from build123d import *

# Parameters (mm, degrees)
SKETCH_1_R               = 87.5
SKETCH_1_R_2             = 70
EXTRUDE_1_DEPTH          = 8
SKETCH_2_R               = 2.75
CUT_EXTRUDE_1_DEPTH      = 10
PATTERN_CIRCULAR_1_COUNT = 4
EXTRUDE_START            = -8
SKETCH_3_R               = 2.75
EXTRUDE_2_DEPTH          = 8
PATTERN_CIRCULAR_2_COUNT = 4
FILLET_1_R               = 10


with BuildPart() as part:
    # 草图1 → 凸台-拉伸1 (new body)
    with BuildSketch(Plane.XY):
        Circle(SKETCH_1_R)
        Circle(SKETCH_1_R_2, mode=Mode.SUBTRACT)
    extrude(amount=EXTRUDE_1_DEPTH)

    # 草图2 → 切除-拉伸1 (cut)
    with BuildSketch(Plane.XY.offset(8)):
        with Locations((42.051550898, 69.52143243)):
            Circle(SKETCH_2_R)
        with Locations((53.351997363, 61.27909005)):
            Circle(SKETCH_2_R)
        with Locations((71.178427561, 39.181551143)):
            Circle(SKETCH_2_R)
        with Locations((15.564640034, 79.745247386)):
            Circle(SKETCH_2_R)
    cut_extrude_1 = extrude(amount=-CUT_EXTRUDE_1_DEPTH, mode=Mode.SUBTRACT)

    # 阵列(圆周)1: 切除-拉伸1 ×4 about axis
    pattern_circular_1_axis = Axis((0, 0, 0), (0, 0, 1))
    for i in range(1, PATTERN_CIRCULAR_1_COUNT):
        add(cut_extrude_1.rotate(pattern_circular_1_axis, i * 360 / PATTERN_CIRCULAR_1_COUNT), mode=Mode.SUBTRACT)

    # 草图3 → 凸台-拉伸2 (add)
    with BuildSketch(Plane.XY.offset(8).offset(EXTRUDE_START)):
        with BuildLine():
            Line((-42.278733745, 76.607823836), (-47.352181794, 85.800762697))
            ThreePointArc((-47.352181794, 85.800762697), (-79.17662028, 57.750002606), (-96.164593228, 18.87779143))
            Line((-96.164593228, 18.87779143), (-85.861243954, 16.85517092))
            ThreePointArc((-85.861243954, 16.85517092), (-70.693410964, 51.562502327), (-42.278733745, 76.607823836))
        make_face()
        with Locations((-89.349607638, 25.800147575)):
            Circle(SKETCH_3_R, mode=Mode.SUBTRACT)
        with Locations((-51.861755237, 77.196880402)):
            Circle(SKETCH_3_R, mode=Mode.SUBTRACT)
        with Locations((-75.136996797, 54.803573902)):
            Circle(SKETCH_3_R, mode=Mode.SUBTRACT)
    extrude_2 = extrude(amount=EXTRUDE_2_DEPTH)

    # 阵列(圆周)2: 凸台-拉伸2 ×4 about axis
    pattern_circular_2_axis = Axis((0, 0, 0), (0, 0, 1))
    for i in range(1, PATTERN_CIRCULAR_2_COUNT):
        add(extrude_2.rotate(pattern_circular_2_axis, i * 360 / PATTERN_CIRCULAR_2_COUNT))

    # 圆角1
    fillet_1_edges = [part.edges().sort_by_distance(p)[0] for p in [
        (-16.85517092, -85.861243954, 4),
        (-76.607823836, -42.278733745, 4),
        (85.861243954, -16.85517092, 4),
        (42.278733745, -76.607823836, 4),
        (16.85517092, 85.861243954, 4),
        (76.607823836, 42.278733745, 4),
        (-85.861243954, 16.85517092, 4),
        (-42.278733745, 76.607823836, 4),
    ]]
    fillet(fillet_1_edges, radius=FILLET_1_R)


solid = part.part
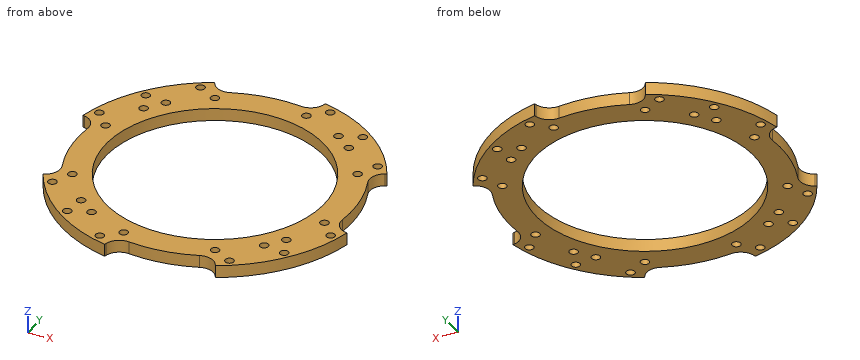
Geometry check sheet. Reference: the model listing, model coordinates, mm. Give positions to 0.01 mm unless a question says otherwise; leave off trailing zeros. Order: outer loops, then holes, each group sorted by start corner. A loop starts at its lowest first (then second) coordinate and runs counter-clockwise, first axis right, second up.
1) Material ranges on probe 1 along Y at (x, z) = (1, 1.75); probe 2 along X at (y, z) = (-50, 4); probe 3 along X at (y, z) = (55.5, 4.25), recorded low to high.
Results are:
probe 1: y = -87.49 to -69.99, 69.99 to 87.49
probe 2: x = -84.29 to -79.22, -75.17 to -48.99, 48.99 to 84.29
probe 3: x = -80.77 to -77.8, -72.48 to -63, -59.56 to -42.66, 42.66 to 80.77
2) Gauge pin test, flat ends, axial feed: pin 1 (4.5 mm diameter, centred on x = -79.75, y = 15.56, fed in from +Z); pin 2 (7 mm diameter, centred on x = -69.52, y = 42.05, fed in from -Z); pin 3 (1.5 mm diameter, centred on x = -75, z = 4.5, fed in from -Y); pin 4 (1 mm diameter, centred on x = 21.5, z = 4, fed in from -Y). Record the tip position at first contact, or that the pin passes through.
Results are:
pin 1: passes through
pin 2: stops at z = 0
pin 3: stops at y = -63.96
pin 4: stops at y = -84.94
3) Cross-section at A-A (x = 0). Record the boundary of the cut face in (y, z), then the cut area to 3 significant figures.
Results are:
outline: (-87.5, 0) - (-70, 0) - (-70, 8) - (-87.5, 8) - close; (70, 0) - (87.5, 0) - (87.5, 8) - (70, 8) - close
area: 280 mm2
4) Cross-section at C-C (z = 6). Give the number of separate pieces and of enclosed holes in the cut face, then the cut area to 3 significant figures.
Results are:
separate pieces: 1
enclosed holes: 29
area: 11,500 mm2
